CAD build for the part. Positions are in the model's coordinates, mm. A direction names the side the tool comes from. Give positions to 0.01 mm unless a question says otherwise; leave off trailing zeros. Loops run counter-clockwise (first coordinate to the right, second up) from the corner with the lowest first, then second, coordinate; pieces in that order, holes last. Notation, with made-up numbers: (34.5, -29) -> (42.5, -29) arc R12 cw to (42.5, -14) -> close; hole circle Ø2 at (85, -35). An arc over 180 degrees is marked (long way). Use one line per item in the form item = value.
```python
from build123d import *

# Parameters (mm, degrees)
CYLINDER015_R            = 3
CYLINDER015_DEPTH        = 4
ARRAY002_COUNT           = 4
ARRAY002_PLACEMENT_ANGLE = 45
CYLINDER014_R            = 4
CYLINDER014_DEPTH        = 10
ARRAY001_Y_COUNT         = 2
ARRAY001_Y_PITCH         = 80
CYLINDER011_R            = 4
CYLINDER011_DEPTH        = 25
CYLINDER012_R            = 11
CYLINDER012_DEPTH        = 10
CYLINDER013_R            = 11
CYLINDER013_DEPTH        = 4
CYLINDER010_R            = 1.5
CYLINDER010_DEPTH        = 25
ARRAY_COUNT              = 4
ARRAY_PLACEMENT_ANGLE    = 45
CYLINDER008_R            = 1.5
CYLINDER008_DEPTH        = 25
CYLINDER007_R            = 1.5
CYLINDER007_DEPTH        = 25
CYLINDER006_R            = 1.5
CYLINDER006_DEPTH        = 25
CYLINDER009_R            = 1.5
CYLINDER009_DEPTH        = 25
CYLINDER003_R            = 2
CYLINDER003_DEPTH        = 25
CYLINDER004_R            = 2
CYLINDER004_DEPTH        = 25
CYLINDER002_R            = 2
CYLINDER002_DEPTH        = 25
CYLINDER001_R            = 2
CYLINDER001_DEPTH        = 25
CYLINDER_R               = 2
CYLINDER_DEPTH           = 25
CYLINDER005_R            = 2
CYLINDER005_DEPTH        = 25
BOX_W                    = 70
BOX_H                    = 350
BOX_DEPTH                = 18


with BuildPart() as array002:
    # Cylinder015 → Cylinder015 (new body)
    with BuildSketch(Plane(origin=(22, 0, 0), x_dir=(1, 0, 0), z_dir=(0, 0, 1))):
        Circle(CYLINDER015_R)
    extrude(amount=CYLINDER015_DEPTH)

    # Array002: Array002 ×4 about axis
    array002_axis = Axis((0, 0, 0), (0, 0, 1))


with BuildPart() as array002_1:
    add(array002.part)
    for i in range(1, ARRAY002_COUNT):
        add(array002.part.rotate(array002_axis, i * 360 / ARRAY002_COUNT))


with BuildPart() as array002_2:
    # Array002 placement: moved
    add(array002_1.part.moved(Location((21, 280, 0))).rotate(Axis((21, 280, 0), (0, 0, 1)), ARRAY002_PLACEMENT_ANGLE))


with BuildPart() as array001:
    # Cylinder014 → Cylinder014 (new body)
    with BuildSketch(Plane.XY):
        Circle(CYLINDER014_R)
    extrude(amount=CYLINDER014_DEPTH)

    # Array001 Y: Array001 ×2


with BuildPart() as array001_1:
    add(array001.part)
    with Locations(*[(0, i * ARRAY001_Y_PITCH, 0) for i in range(1, ARRAY001_Y_COUNT)]):
        add(array001.part)


with BuildPart() as array001_2:
    # Array001 placement: moved
    add(array001_1.part.moved(Location((21, 240, 0))))


with BuildPart() as cilindro011:
    # Cylinder011 → Cylinder011 (new body)
    with BuildSketch(Plane.XY):
        Circle(CYLINDER011_R)
    extrude(amount=CYLINDER011_DEPTH)


with BuildPart() as cilindro012:
    # Cylinder012 → Cylinder012 (new body)
    with BuildSketch(Plane.XY.offset(15)):
        Circle(CYLINDER012_R)
    extrude(amount=CYLINDER012_DEPTH)


with BuildPart() as fusion002:
    # Cylinder013 → Cylinder013 (new body)
    with BuildSketch(Plane.XY):
        Circle(CYLINDER013_R)
    extrude(amount=CYLINDER013_DEPTH)

    # Fusion002: union Cilindro011, Cilindro012
    add(cilindro011.part)
    add(cilindro012.part)


with BuildPart() as fusion002_1:
    # Fusion002 placement: moved
    add(fusion002.part.moved(Location((21, 280, 0))))


with BuildPart() as array:
    # Cylinder010 → Cylinder010 (new body)
    with BuildSketch(Plane(origin=(22, 0, 0), x_dir=(1, 0, 0), z_dir=(0, 0, 1))):
        Circle(CYLINDER010_R)
    extrude(amount=CYLINDER010_DEPTH)

    # Array: Array ×4 about axis
    array_axis = Axis((0, 0, 0), (0, 0, 1))


with BuildPart() as array_1:
    add(array.part)
    for i in range(1, ARRAY_COUNT):
        add(array.part.rotate(array_axis, i * 360 / ARRAY_COUNT))


with BuildPart() as array_2:
    # Array placement: moved
    add(array_1.part.moved(Location((21, 280, 0))).rotate(Axis((21, 280, 0), (0, 0, 1)), ARRAY_PLACEMENT_ANGLE))


with BuildPart() as cilindro008:
    # Cylinder008 → Cylinder008 (new body)
    with BuildSketch(Plane(origin=(6, 185, 0), x_dir=(1, 0, 0), z_dir=(0, 0, 1))):
        Circle(CYLINDER008_R)
    extrude(amount=CYLINDER008_DEPTH)


with BuildPart() as cilindro007:
    # Cylinder007 → Cylinder007 (new body)
    with BuildSketch(Plane(origin=(6, 136, 0), x_dir=(1, 0, 0), z_dir=(0, 0, 1))):
        Circle(CYLINDER007_R)
    extrude(amount=CYLINDER007_DEPTH)


with BuildPart() as cilindro006:
    # Cylinder006 → Cylinder006 (new body)
    with BuildSketch(Plane(origin=(64, 136, 0), x_dir=(1, 0, 0), z_dir=(0, 0, 1))):
        Circle(CYLINDER006_R)
    extrude(amount=CYLINDER006_DEPTH)


with BuildPart() as fusion001:
    # Cylinder009 → Cylinder009 (new body)
    with BuildSketch(Plane(origin=(64, 185, 0), x_dir=(1, 0, 0), z_dir=(0, 0, 1))):
        Circle(CYLINDER009_R)
    extrude(amount=CYLINDER009_DEPTH)

    # Fusion001: union Cilindro008, Cilindro007, Cilindro006
    add(cilindro008.part)
    add(cilindro007.part)
    add(cilindro006.part)


with BuildPart() as cilindro003:
    # Cylinder003 → Cylinder003 (new body)
    with BuildSketch(Plane(origin=(60, 50, 0), x_dir=(1, 0, 0), z_dir=(0, 0, 1))):
        Circle(CYLINDER003_R)
    extrude(amount=CYLINDER003_DEPTH)


with BuildPart() as cilindro004:
    # Cylinder004 → Cylinder004 (new body)
    with BuildSketch(Plane(origin=(12, 35, 0), x_dir=(1, 0, 0), z_dir=(0, 0, 1))):
        Circle(CYLINDER004_R)
    extrude(amount=CYLINDER004_DEPTH)


with BuildPart() as cilindro002:
    # Cylinder002 → Cylinder002 (new body)
    with BuildSketch(Plane(origin=(10, 50, 0), x_dir=(1, 0, 0), z_dir=(0, 0, 1))):
        Circle(CYLINDER002_R)
    extrude(amount=CYLINDER002_DEPTH)


with BuildPart() as cilindro001:
    # Cylinder001 → Cylinder001 (new body)
    with BuildSketch(Plane(origin=(60, 20, 0), x_dir=(1, 0, 0), z_dir=(0, 0, 1))):
        Circle(CYLINDER001_R)
    extrude(amount=CYLINDER001_DEPTH)


with BuildPart() as cilindro:
    # Cylinder → Cylinder (new body)
    with BuildSketch(Plane(origin=(10, 20, 0), x_dir=(1, 0, 0), z_dir=(0, 0, 1))):
        Circle(CYLINDER_R)
    extrude(amount=CYLINDER_DEPTH)


with BuildPart() as fusion:
    # Cylinder005 → Cylinder005 (new body)
    with BuildSketch(Plane(origin=(26.5, 35, 0), x_dir=(1, 0, 0), z_dir=(0, 0, 1))):
        Circle(CYLINDER005_R)
    extrude(amount=CYLINDER005_DEPTH)

    # Fusion: union Cilindro003, Cilindro004, Cilindro002, Cilindro001, Cilindro
    add(cilindro003.part)
    add(cilindro004.part)
    add(cilindro002.part)
    add(cilindro001.part)
    add(cilindro.part)


with BuildPart() as cut005:
    # Box → Box (new body)
    with BuildSketch(Plane.XY):
        with Locations((35, 175)):
            Rectangle(BOX_W, BOX_H)
    extrude(amount=BOX_DEPTH)

    # Cut: cut Fusion
    add(fusion.part, mode=Mode.SUBTRACT)

    # Cut001: cut Fusion001
    add(fusion001.part, mode=Mode.SUBTRACT)

    # Cut002: cut Array
    add(array_2.part, mode=Mode.SUBTRACT)

    # Cut003: cut Fusion002
    add(fusion002_1.part, mode=Mode.SUBTRACT)

    # Cut004: cut Array001
    add(array001_2.part, mode=Mode.SUBTRACT)

    # Cut005: cut Array002
    add(array002_2.part, mode=Mode.SUBTRACT)


solid = cut005.part
```
1. Drill centre lines: line 1 (Y direction, x = 21, z = 2.5); line 2 (X direction, y = 34, z = 3.75); line 3 (Y direction, x = 5, z = 4.5). Where is each one in solid material? Low to high.
Result sheet:
line_1 = 0 to 236, 244 to 269, 291 to 316, 324 to 350
line_2 = 0 to 10.27, 13.73 to 24.77, 28.23 to 70
line_3 = 0 to 134.88, 137.12 to 183.88, 186.12 to 263.01, 265.88 to 294.12, 296.99 to 350
2. Mould opens along X. For faces 4 (the cylindrical face through (19.568, 290.906, 1.972)), 5 (the flat face through (70, 173, 9)), 6 (the flat face through (35, 177, 0)), 7 (the flat face through (21, 320, 10)) say: pulls with the +X half, pulls with the -X half, needs draft (parallel to the pull), parting line crosses it, or undercut.
Result sheet:
face_4 = undercut
face_5 = pulls with the +X half
face_6 = needs draft
face_7 = undercut
3. Cut at A-A, the plane x = 21. Write the cut outline in (y, z).
Result sheet:
outline = (0, 0) -> (236, 0) -> (236, 10) -> (244, 10) -> (244, 0) -> (269, 0) -> (269, 4) -> (276, 4) -> (276, 15) -> (269, 15) -> (269, 18) -> (0, 18) -> close; (284, 4) -> (291, 4) -> (291, 0) -> (316, 0) -> (316, 10) -> (324, 10) -> (324, 0) -> (350, 0) -> (350, 18) -> (291, 18) -> (291, 15) -> (284, 15) -> close
4. Cut at B-B, the plane y = 280. Write the cut outline in (x, z).
Result sheet:
outline = (0, 0) -> (10, 0) -> (10, 4) -> (17, 4) -> (17, 15) -> (10, 15) -> (10, 18) -> (0, 18) -> close; (25, 4) -> (32, 4) -> (32, 0) -> (70, 0) -> (70, 18) -> (32, 18) -> (32, 15) -> (25, 15) -> close
5. Drop a flat-ended pin along its axis: P1, Ø11, axis at x = 19, y = 280.5, coming from the -Z side. Give the stop position or say it passes through.
Result sheet:
P1 = 4
6. Tool access for faces 1 (the flat face through (35, 350, 9)), 2 (the cylindrical face through (19.568, 290.906, 16.479)), 3 (the flat face through (36, 294, 4)): list every direction of +Z, -Z, +X, -X, +Y, -Y with a clear straight run to the whole face (end or side of a thin tool).
Result sheet:
face_1 = +Z, -Z, +X, -X, +Y
face_2 = +Z
face_3 = -Z
